Design review of the part shown in the three views and the two pictorial views. Dimensions are in mm from the part's minimum x, y and z. A direction names the side the tool comes from. Coordinates: 2 decimals unless noted, no trailing zeros. Write each loop counter-clockwise with the first axis right and the second up, starting at its lowest first coordinate (ties: lowest second). Pieces come first, ordered by that corner, then holes. Notation, with made-up numbers: (6, 20) -> (21, 20) arc R31 ccw to (21, 56) -> close; hole circle Ø3 at (26, 21.5). An arc over 180 degrees is marked (long way). Answer in a Markdown table with one row per item. Add a question column.
Item 1: Draft analysis for pull direction Y (two halves, no side actions). For the marked faces 4, 5 and 6, state which applies: released by +Y, released by -Y, zero draft, split by the parting line, or undercut.
Item 2: Take a section at C-C, the plane y = 14.25. Write out the cut boundary in (x, z), and give its area (3 significant figures).
Item 3: Take a section at A-A, the plane z = 3. Write out the cut boundary in (x, y), and give its area (3 significant figures).
Item 4: Take a section at B-B, the plane x = 4.1. Write out the cut boundary in (y, z) (3 decimals).
Item 5: To check wall thickness, follow line 1 (Y direction, x = 5.1, z = 2.55); line 2 (Z direction, x = 3, y = 7.5); line 3 (Y direction, x = 0.5, z = 3.6). State the ranges of each line that lie inside material, in increasing order.
Item 6: Take a section at D-D, the plane y = 23.25. Write out the cut boundary in (x, z).
Item 7: For the marked faces 1, 2 and 3, list the 3-axis set-ups (+Z, -Z, +X, -X, +Y, -Y) from which the entire face can be reached by the end or side of a thin tool; tool diameter is ignored.
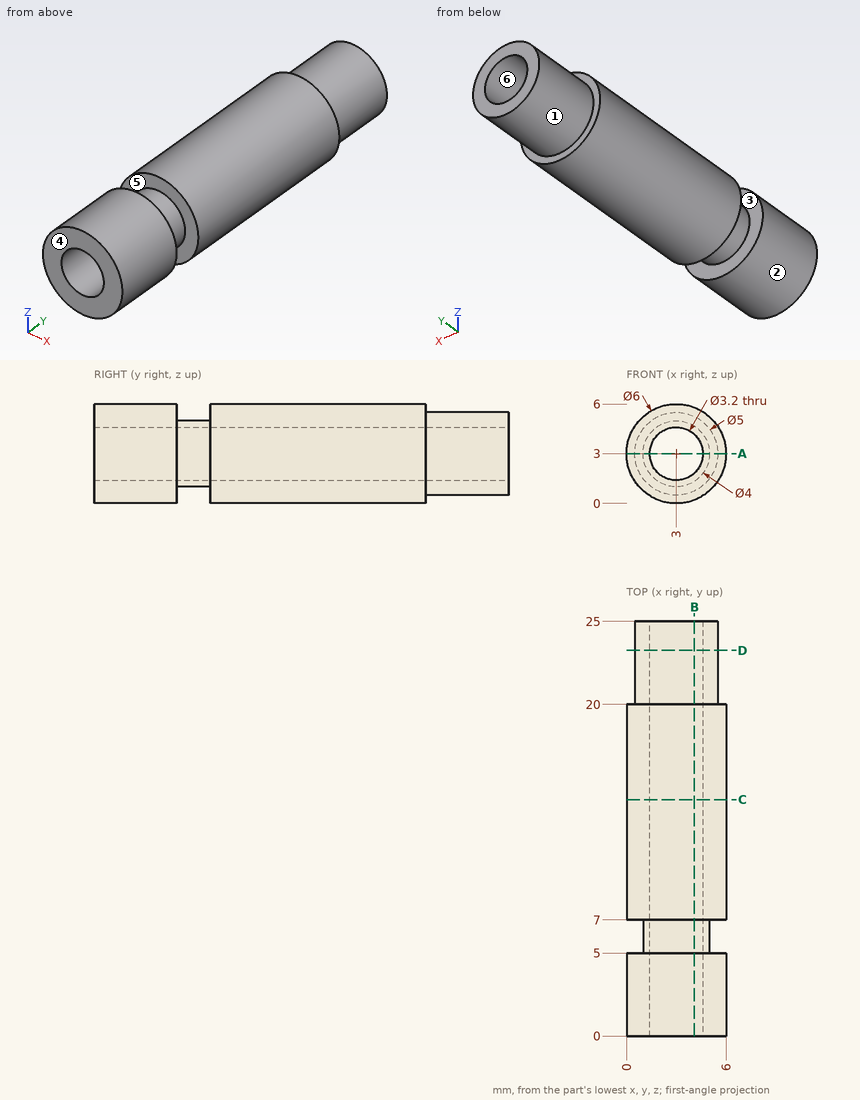
Answers:
| question | item | result |
|---|---|---|
| 1 | face 4 | released by -Y |
| 1 | face 5 | undercut |
| 1 | face 6 | zero draft |
| 2 | outline | circle Ø6 at (3, 3); hole circle Ø3.2 at (3, 3) |
| 2 | area | 20.2 mm^2 |
| 3 | outline | (0, 0) -> (1.4, 0) -> (1.4, 25) -> (0.5, 25) -> (0.5, 20) -> (0, 20) -> (0, 7) -> (1, 7) -> (1, 5) -> (0, 5) -> close; (4.6, 0) -> (6, 0) -> (6, 5) -> (5, 5) -> (5, 7) -> (6, 7) -> (6, 20) -> (5.5, 20) -> (5.5, 25) -> (4.6, 25) -> close |
| 3 | area | 61.0 mm^2 |
| 4 | outline | (0, 0.209) -> (5, 0.209) -> (5, 1.33) -> (7, 1.33) -> (7, 0.209) -> (20, 0.209) -> (20, 0.755) -> (25, 0.755) -> (25, 1.838) -> (0, 1.838) -> close; (0, 4.162) -> (25, 4.162) -> (25, 5.245) -> (20, 5.245) -> (20, 5.791) -> (7, 5.791) -> (7, 4.67) -> (5, 4.67) -> (5, 5.791) -> (0, 5.791) -> close |
| 5 | line 1 | y = 0 to 5, 7 to 25 |
| 5 | line 2 | z = 0 to 1.4, 4.6 to 6 |
| 5 | line 3 | y = 0 to 5, 7 to 20 |
| 6 | outline | circle Ø5 at (3, 3); hole circle Ø3.2 at (3, 3) |
| 7 | face 1 | +Y |
| 7 | face 2 | +Y, -Y |
| 7 | face 3 | none |
